Input: part model. Units: mm. Frame: model coordinates. Face numbers are marked on the shaded views. A direction names the side the tool comes from. Round coordinates to 2 decimals unless told otherwise and drop trailing zeros. Order: outer loops, then holes, each group sorted by start corner. A loop starts at its lowest first (then second) coordinate and runs counter-clockwise, first axis right, second up. Notation, with made-up numbers: (46.5, 80.25) - (53.5, 80.25) arc R8 ccw to (53.5, 85.25) - close; hole circle Ø6 at (16, 67.5). An arc over 180 degrees is marked (long way). One line per item, written item: value. Start each with the question number.
from build123d import *

# Parameters (mm, degrees)
SKETCH1_R               = 11
SKETCH1_R_2             = 7
EXTRUDE2_DEPTH          = 32
SKETCH_R                = 14
EXTRUDE3_DEPTH          = 22
FILLET1_R               = 20
SKETCH5_R               = 2.75
EXTRUDE5_DEPTH          = 10
CIRPATTERN1_COUNT       = 3
CIRPATTERN1_ANGLE       = 90
MIRROR1_COPY_1_SKETCH_R = 2.75
MIRROR1_COPY_1_DEPTH    = 10
MIRROR1_COPY_2_SKETCH_R = 2.75
MIRROR1_COPY_2_DEPTH    = 10
EXTRUDE10_START         = 14.5
EXTRUDE10_OUTLINE_R     = 8
EXTRUDE10_OUTLINE_R_2   = 7
EXTRUDE10_DEPTH         = 3
EXTRUDE11_START         = 45.358117006
EXTRUDE11_OUTLINE_R     = 1.5
EXTRUDE11_DEPTH         = 8.141882994
M5_CLEARANCE_HOLE1_D    = 5.5


# Read off the part's stored shape, not the designer's step: Extrude10, Extrude11
with BuildPart() as part:
    # Sketch1 → Extrude2 (new body)
    with BuildSketch(Plane(origin=(0, 0, 0), x_dir=(1, 0, 0), z_dir=(0, 1, 0))):
        with BuildLine():
            Line((-15, -35), (15, -35))
            Line((15, -35), (46.596913018, -13.162301226))
            ThreePointArc((46.596913018, -13.162301226), (53.5, 0), (46.596913018, 13.162301226))
            Line((46.596913018, 13.162301226), (15, 35))
            Line((15, 35), (-15, 35))
            Line((-15, 35), (-46.596913018, 13.162301226))
            ThreePointArc((-46.596913018, 13.162301226), (-53.5, 0), (-46.596913018, -13.162301226))
            Line((-46.596913018, -13.162301226), (-15, -35))
        make_face()
        with Locations(Location((-37.5, 0, 0), (0, 0, 270))):
            Circle(SKETCH1_R, mode=Mode.SUBTRACT)
        with Locations(Location((37.5, 0, 0), (0, 0, 270))):
            Circle(SKETCH1_R_2, mode=Mode.SUBTRACT)
        with BuildLine():
            Line((-20, 13.266499161), (-20, -13.266499161))
            ThreePointArc((-20, -13.266499161), (0, -24), (20, -13.266499161))
            Line((20, -13.266499161), (20, 13.266499161))
            ThreePointArc((20, 13.266499161), (0, 24), (-20, 13.266499161))
        make_face(mode=Mode.SUBTRACT)
    extrude(amount=EXTRUDE2_DEPTH)

    # Sketch → Extrude3 (add)
    with BuildSketch(Plane(origin=(0, 0, 0), x_dir=(1, 0, 0), z_dir=(0, 1, 0))):
        with BuildLine():
            Line((20, 13.266499161), (20, -13.266499161))
            ThreePointArc((20, -13.266499161), (0, -24), (-20, -13.266499161))
            Line((-20, -13.266499161), (-20, 13.266499161))
            ThreePointArc((-20, 13.266499161), (0, 24), (20, 13.266499161))
        make_face()
        with Locations(Location((0, 0, 0), (0, 0, 90))):
            Circle(SKETCH_R, mode=Mode.SUBTRACT)
    extrude(amount=EXTRUDE3_DEPTH)

    # Fillet1
    fillet1_edges = [part.edges().sort_by_distance(p)[0] for p in [
        (15, 16, 35),
        (-15, 16, 35),
        (-15, 16, -35),
        (15, 16, -35),
    ]]
    fillet(fillet1_edges, radius=FILLET1_R)

    # Sketch5 → Extrude5 (add)
    with BuildSketch(Plane(origin=(0, 22, 0), x_dir=(1, 0, 0), z_dir=(0, 1, 0))):
        with Locations(Location((13.435028843, 13.435028843, 0), (0, 0, 90))):
            Circle(SKETCH5_R)
    extrude5 = extrude(amount=EXTRUDE5_DEPTH)

    # CirPattern1: Extrude5 ×3 about axis
    cirpattern1_axis = Axis((0, 0, 0), (0, 1, 0))
    for i in range(1, CIRPATTERN1_COUNT):
        add(extrude5.rotate(cirpattern1_axis, i * CIRPATTERN1_ANGLE / (CIRPATTERN1_COUNT - 1)))

    # Mirror1: Extrude5 across plane
    add(extrude5.mirror(Plane.XY))

    # Mirror1 copy 1 sketch → Mirror1 copy 1 (add)
    with BuildSketch(Plane(origin=(0, 22, 0), x_dir=(0.7071067811865467, 0, 0.7071067811865483), z_dir=(0, 1, 0))):
        with Locations((13.435028843, -13.435028843)):
            Circle(MIRROR1_COPY_1_SKETCH_R)
    extrude(amount=MIRROR1_COPY_1_DEPTH)

    # Mirror1 copy 2 sketch → Mirror1 copy 2 (add)
    with BuildSketch(Plane.ZX.offset(22)):
        with Locations((13.435028843, -13.435028843)):
            Circle(MIRROR1_COPY_2_SKETCH_R)
    extrude(amount=MIRROR1_COPY_2_DEPTH)

    # Extrude10 outline → Extrude10 (cut)
    with BuildSketch(Plane(origin=(0, 0, 0), x_dir=(1, 0, 0), z_dir=(0, 1, 0)).offset(EXTRUDE10_START)):
        with Locations((37.5, 0)):
            Circle(EXTRUDE10_OUTLINE_R)
        with Locations((37.5, 0)):
            Circle(EXTRUDE10_OUTLINE_R_2, mode=Mode.SUBTRACT)
    extrude(amount=EXTRUDE10_DEPTH, mode=Mode.SUBTRACT)

    # Extrude11 outline → Extrude11 (cut)
    with BuildSketch(Plane.YZ.offset(EXTRUDE11_START)):
        with Locations((16, 0)):
            Circle(EXTRUDE11_OUTLINE_R)
    extrude(amount=EXTRUDE11_DEPTH, mode=Mode.SUBTRACT)

    # M5 Clearance Hole1 (through all)
    with Locations(Plane(origin=(0, 32, 0), x_dir=(1, 0, 0), z_dir=(0, 1, 0))):
        with Locations((0, 28), (0, -28)):
            Hole(M5_CLEARANCE_HOLE1_D / 2)


solid = part.part
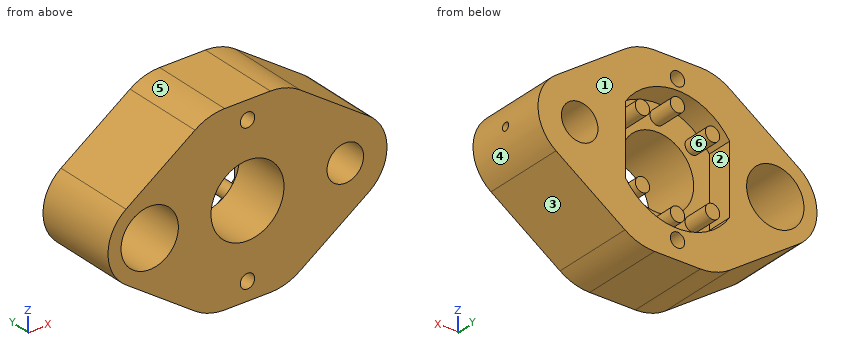
Item 1: Reachability of the marked faces 1 and 2 from +Z, -Z, +X, -X, +Y, -Y: full face, straight path, thin tool, end or side. Return the list, or none.
Item 2: Section query B-B on x = -39.5. Return loops of the section in (y, z), and give its area (3 significant figures).
Item 3: Line query: L1, parallel to X at y = 5, z = 0; L2, parallel to X at y = 15.5, z = 0; L3, parallel to Z at x = -13.5, y = 23.5. Output: solid intervals per line, ascending.
Item 4: Section query A-A on y = 26.5. Give the number of separate pieces and of enclosed holes in the cut face, and give its area (3 significant figures).
Item 5: Section query D-D on x = 0. Return loops of the section in (y, z).
Item 6: Section query C-C on z = 28. Return loops of the section in (x, y), and give its area (3 significant figures).
Item 7: Pull-direction query (Z, two-part tool) for the marked faces 3, 4, 5 and 6; classes: released by +Z, released by -Z, zero draft, split by the parting line, or undercut.
Item 8: First-contact query: pin 1 Ø17 at (x, z) = (0, 0) entering from -Y; pin 2 Ø6 at (y, z) = (8.5, 9) entering from +X; pin 3 Ø5 at (x, y) = (38, 7) entering from +Z; pin 4 Ø3 at (y, z) = (22.5, 4) entering from -X. Flat tips, straight axial feed; report the tip coordinate or a pass-through.
Geometry results:
1. face 1: +Z, -Z, +X, -X, +Y
1. face 2: +Y
2. outline: (0, -18.07) - (32, -18.07) - (32, -10.82) - (0, -10.82) - close; (0, 10.82) - (32, 10.82) - (32, 18.07) - (0, 18.07) - close
2. area: 464 mm^2
3. L1: x = -53.5 to -48.5, -26.5 to -14, 14 to 30.5, 44.5 to 53.5
3. L2: x = -53.5 to -48.5, -26.5 to -14, 14 to 29.5
3. L3: z = -34.43 to -19.84, -16.18 to -10.69, 10.69 to 16.18, 19.84 to 34.43
4. separate pieces: 7
4. enclosed holes: 5
4. area: 3,280 mm^2
5. outline: (0, -35) - (32, -35) - (32, -30.75) - (0, -30.75) - close; (0, -25.25) - (32, -25.25) - (32, -24) - (22, -24) - (22, -21.75) - (32, -21.75) - (32, -16.25) - (22, -16.25) - (22, -14) - (0, -14) - close; (0, 14) - (22, 14) - (22, 16.25) - (32, 16.25) - (32, 21.75) - (22, 21.75) - (22, 24) - (32, 24) - (32, 25.25) - (0, 25.25) - close; (0, 30.75) - (32, 30.75) - (32, 35) - (0, 35) - close
6. outline: (-25.13, 0) - (-2.75, 0) - (-2.75, 32) - (-25.13, 32) - close; (2.75, 0) - (25.13, 0) - (25.13, 32) - (2.75, 32) - close
6. area: 1,430 mm^2
7. face 3: released by -Z
7. face 4: split by the parting line
7. face 5: released by +Z
7. face 6: undercut
8. pin 1: passes through
8. pin 2: stops at x = 52.33
8. pin 3: stops at z = 20.83
8. pin 4: stops at x = -53.3
